Source: three-view drawing plus pictorial views. Frame: mm from the lowest corner of the part. A direction names the side the tool comes from. Give positions to 0.01 mm unless a question says otherwise; leave off trailing zeros. Loops run counter-clockwise (first coordinate to the right, second up) from the corner with the lowest first, then second, coordinate; pieces in that order, holes last. Notation, with made-up numbers: M 33.5,-22 L 64.5,-22 A21 cw 64.5,-8 Z; hole C 38,-38 d5. An arc over 180 degrees is marked long. Answer as a JSON object with one key per item and string values. Group by question number.
1) Section query C-C on x = 14.5. Return loops of the section in (y, z).
2) Access query for the marked faces 1, 2 and 3. Directions: +Z, -Z, +X, -X, +Y, -Y. A direction counts if a zero-diameter tool reaches every point of the face in a straight line with its end or side. Return the directions, or none.
3) Section query A-A on z = 33. Return loops of the section in (x, y).
4) Section query B-B on z = 7. Return loops of the section in (x, y).
5) Section query D-D on y = 13. Return loops of the section in (x, z), plus the area to 3 significant figures.
6) Draft query along Y for the marked faces 4, 5, 6 and 7. Return one class per face: +Y half, -Y half, draft (parallel to the pull), parting line (faces both ways), or undercut.
7) Ray query, L1, parallel to Y at x = 35, z = 58; L2, parallel to Z at x = 8.5, y = 15; L3, parallel to Y at x = 41, z = 7.5. Return the intervals inside material, ascending.
8) First-contact query: P1, Ø12, axis at x = 36, y = 50, coming from the +Z side; P2, Ø4, axis at x = 34.5, z = 23, coming from the +Y side; P3, Ø3, axis at x = 6.5, y = 43, coming from the +Z side; P4, Ø5, axis at y = 47.5, z = 39, coming from the -X side. Flat tips, straight axial feed; report the tip coordinate or a pass-through.
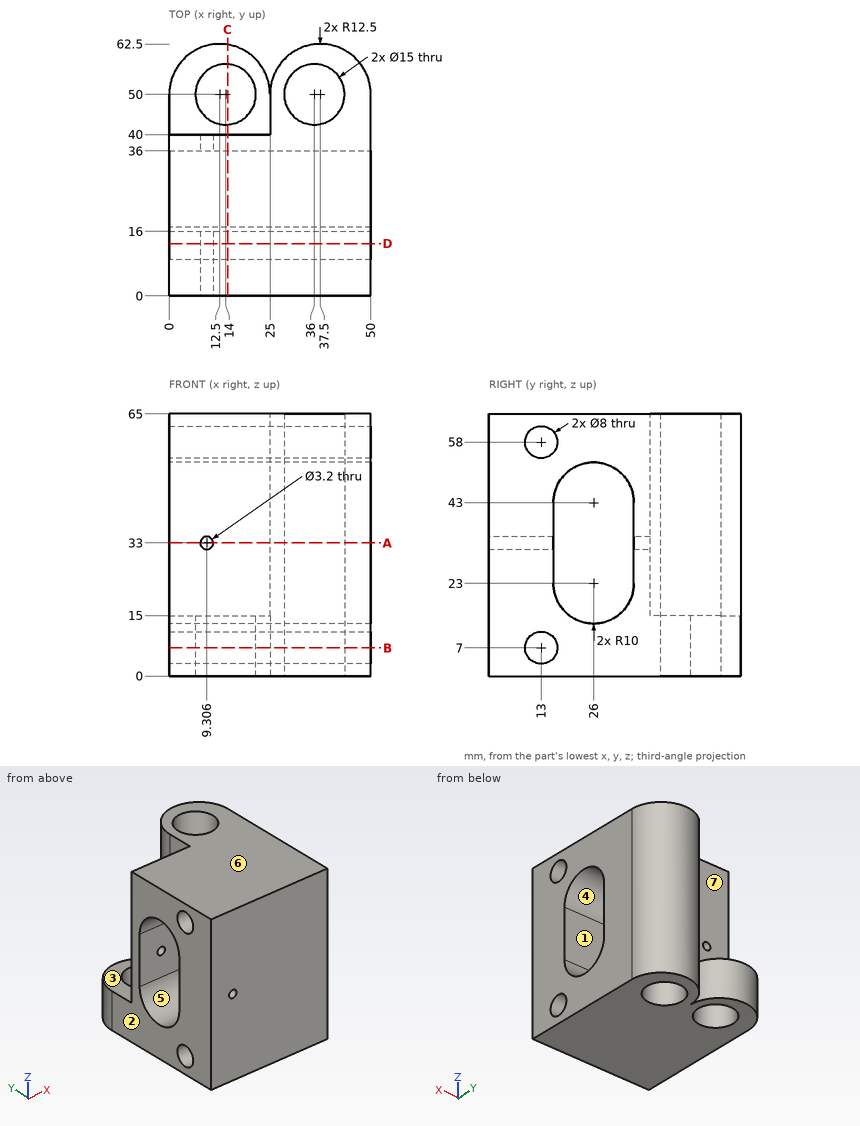
Output:
{
 "1": {"outline": "M 0,0 L 42.52,0 L 42.52,15 L 40,15 L 40,65 L 0,65 Z; M 57.48,0 L 62.34,0 L 62.34,15 L 57.48,15 Z; hole C 13,7 d8; hole C 13,58 d8; hole M 16,23 A10 ccw 36,23 L 36,43 A10 ccw 16,43 Z"},
 "2": {"face 1": "+X, -X", "face 2": "+Z, -Z, -X, +Y, -Y", "face 3": "+Z, -X, +Y"},
 "3": {"outline": "M 0,0 L 7.71,0 L 7.71,16 L 0,16 Z; M 0,36 L 7.71,36 L 7.71,40 L 0,40 Z; M 10.91,0 L 50,0 L 50,16 L 10.91,16 Z; M 10.91,36 L 50,36 L 50,50 A12.5 ccw 25,50 L 25,40 L 10.91,40 Z; hole C 36,50 d15"},
 "4": {"outline": "M 0,0 L 50,0 L 50,9 L 0,9 Z; M 0,17 L 50,17 L 50,50 A12.5 ccw 25,50 A12.5 ccw 0,50 Z; hole C 14,50 d15; hole C 36,50 d15"},
 "5": {"outline": "M 0,0 L 50,0 L 50,3 L 0,3 Z; M 0,11 L 50,11 L 50,54 L 0,54 Z; M 0,62 L 50,62 L 50,65 L 0,65 Z; hole C 9.31,33 d3.2", "area": "2,440 mm^2"},
 "6": {"face 4": "undercut", "face 5": "undercut", "face 6": "draft", "face 7": "+Y half"},
 "7": {"L1": "y = 0 to 9, 17 to 42.57, 57.43 to 62.25", "L2": "z = 0 to 3.54, 10.46 to 31.62, 34.38 to 54.54, 61.46 to 65", "L3": "y = 0 to 9.03, 16.97 to 44.41, 55.59 to 62"},
 "8": {"P1": "passes through", "P2": "stops at y = 62.46", "P3": "stops at z = 15", "P4": "stops at x = 25"}
}
